Can you work these out from the model? Positions are in its coordinate system, mm. A direction names the side the tool comes from. Give positions to 0.01 mm unless a question says otherwise; leave off trailing zeros. Write each loop counter-clockwise with the first axis right and the second up, starting at its lowest first coordinate (ties: lowest second). Pieces come first, ordered by that corner, then holes.
1. If I drill on probe 1 along X at (y, z) = (1.2, 58); probe 2 along Z at (x, y) = (-8, 2.4); probe 3 along Z at (x, y) = (41, 1.75), over which ranges is the centre line in solid material (lowest first)?
2. Suppose I cut it at A-A (x = 39). Please give me the cut outline in (y, z) (3 decimals).
3. Suppose I cut it at B-B (y = 2). Give the number of separate pieces and of enclosed holes in the cut face, and give its area (3 significant figures).
4. Suppose I cut it at C-C (z = 26). Please give me the cut outline in (x, y) (3 decimals).
5. On a 3-axis mill with a long thin cutter (end or side, diameter ignored), from which of +Z, -Z, +X, -X, +Y, -Y can I reach the whole of each face in a straight line? I mean faces 1 (the cylindrical face through (0.71, 1.565, 124.636)), 2 (the flat face through (-97.4, 1.6, 23.5)), 3 (the flat face through (97.94, 1.57, 23.25)), 4 (the flat face through (91.042, 1.565, 82.953)), 5 (the cylindrical face through (118.74, 1.61, 1.81)). Say none if no direction works.
6. I'm going to push flat-ended pins straight in: pin 1 (1 mm diameter, centred on y = 2.5, z = 50.5, fed in from -X); pin 2 (4 mm diameter, centred on x = -61.5, z = 40, fed in from -Y); pin 3 (1 mm diameter, centred on x = 36.5, y = 1, fed in from +Z). Where does each tip first touch, or does it pass through?
7. Suppose I cut it at D-D (x = -33). Please give me the cut outline in (y, z) (3 decimals), and give its area (3 significant figures).
8. Thinking about a two-plate mould opening in Z: for faces 6 (the flat face through (-41.28, 1.57, 87.93)), 7 (the flat face through (18, 3.175, 76)), 8 (the cylindrical face through (118.84, 1.61, 131.44)), 9 (the cylindrical face through (-118.74, 1.61, 1.81)), which applies, pulls with the +Z half, pulls with the -Z half, needs draft (parallel to the pull), parting line crosses it, or undercut?
```python
from build123d import *

# Parameters (mm, degrees)
BOSS_EXTRUDE1_DEPTH = 3.175
FILLET1_R           = 6.35
FILLET2_R           = 6.35


with BuildPart() as part:
    # Sketch1 → Boss-Extrude1 (new body)
    with BuildSketch(Plane(origin=(0, 0, 0), x_dir=(1, 0, 0), z_dir=(0, 1, 0))):
        with BuildLine():
            Line((-120.65, 0), (120.65, 0))
            Line((120.65, 0), (120.65, -12.7))
            Line((120.65, -12.7), (65.976752043, -38.1))
            Line((65.976752043, -38.1), (120.65, -63.5))
            Line((120.65, -63.5), (120.65, -76.2))
            Line((120.65, -76.2), (79.645064032, -95.25))
            Line((79.645064032, -95.25), (120.65, -114.3))
            Line((120.65, -114.3), (120.65, -133.35))
            Line((120.65, -133.35), (50.8, -133.35))
            ThreePointArc((50.8, -133.35), (0, -124.634097937), (-50.8, -133.35))
            Line((-50.8, -133.35), (-120.65, -133.35))
            Line((-120.65, -133.35), (-120.65, -114.3))
            Line((-120.65, -114.3), (-79.645064032, -95.25))
            Line((-79.645064032, -95.25), (-120.65, -76.2))
            Line((-120.65, -76.2), (-120.65, -63.5))
            Line((-120.65, -63.5), (-65.976752043, -38.1))
            Line((-65.976752043, -38.1), (-120.65, -12.7))
            Line((-120.65, -12.7), (-120.65, 0))
        make_face()
        Polygon((-111.711303819, -6.35), (111.711303819, -6.35), (0, -58.248638237), align=None, mode=Mode.SUBTRACT)
        Polygon((-58.441082652, -41.600907842), (-119.246973209, -69.85), (-72.109394642, -91.749092158), (-11.303504085, -63.5), align=None, mode=Mode.SUBTRACT)
        Polygon((11.303504085, -63.5), (58.441082652, -41.600907842), (119.246973209, -69.85), (72.109394642, -91.749092158), align=None, mode=Mode.SUBTRACT)
        with BuildLine():
            Line((-104.877147824, -117.475), (0, -68.751361763))
            Line((0, -68.751361763), (104.877147824, -117.475))
            Line((104.877147824, -117.475), (62.737522787, -117.475))
            ThreePointArc((62.737522787, -117.475), (0, -105.584097937), (-62.737522787, -117.475))
            Line((-62.737522787, -117.475), (-104.877147824, -117.475))
        make_face(mode=Mode.SUBTRACT)
    extrude(amount=BOSS_EXTRUDE1_DEPTH)

    # Fillet1
    fillet1_edges = [part.edges().sort_by_distance(p)[0] for p in [
        (104.877147824, 1.5875, 117.475),
        (0, 1.5875, 68.751361763),
        (-104.877147824, 1.5875, 117.475),
        (-62.737522787, 1.5875, 117.475),
        (-111.711303819, 1.5875, 6.35),
        (0, 1.5875, 58.248638237),
        (111.711303819, 1.5875, 6.35),
        (-11.303504085, 1.5875, 63.5),
        (-58.441082652, 1.5875, 41.600907842),
        (-119.246973209, 1.5875, 69.85),
        (-72.109394642, 1.5875, 91.749092158),
        (11.303504085, 1.5875, 63.5),
        (72.109394642, 1.5875, 91.749092158),
        (119.246973209, 1.5875, 69.85),
        (58.441082652, 1.5875, 41.600907842),
    ]]
    fillet(fillet1_edges, radius=FILLET1_R)

    # Fillet2
    fillet2_edges = [part.edges().sort_by_distance(p)[0] for p in [
        (120.65, 1.5875, 12.7),
        (65.976752043, 1.5875, 38.1),
        (120.65, 1.5875, 63.5),
        (120.65, 1.5875, 76.2),
        (79.645064032, 1.5875, 95.25),
        (120.65, 1.5875, 114.3),
        (120.65, 1.5875, 133.35),
        (50.8, 1.5875, 133.35),
        (-50.8, 1.5875, 133.35),
        (-120.65, 1.5875, 133.35),
        (-120.65, 1.5875, 114.3),
        (-79.645064032, 1.5875, 95.25),
        (-120.65, 1.5875, 76.2),
        (-120.65, 1.5875, 63.5),
        (-65.976752043, 1.5875, 38.1),
        (-120.65, 1.5875, 12.7),
        (-120.65, 1.5875, 0),
        (120.65, 1.5875, 0),
    ]]
    fillet(fillet2_edges, radius=FILLET2_R)


solid = part.part
```
Checks:
1. probe 1: x = -108.81 to -93.74, -23.2 to 23.2, 93.74 to 108.81
1. probe 2: z = 0 to 6.35, 54.53 to 72.47, 105.77 to 124.84
1. probe 3: z = 0 to 6.35, 39.2 to 49.7, 77.3 to 87.8, 110.56 to 130.25
2. outline: (0, 0) - (3.175, 0) - (3.175, 6.35) - (0, 6.35) - close; (0, 40.13) - (3.175, 40.13) - (3.175, 50.633) - (0, 50.633) - close; (0, 76.367) - (3.175, 76.367) - (3.175, 86.87) - (0, 86.87) - close; (0, 110.079) - (3.175, 110.079) - (3.175, 129.709) - (0, 129.709) - close
3. separate pieces: 1
3. enclosed holes: 4
3. area: 12,800 mm2
4. outline: (-92.022, 0) - (-69.415, 0) - (-69.415, 3.175) - (-92.022, 3.175) - close; (69.415, 0) - (92.022, 0) - (92.022, 3.175) - (69.415, 3.175) - close
5. face 1: +Z, +Y, -Y
5. face 2: -X, +Y, -Y
5. face 3: +X, +Y, -Y
5. face 4: +Y, -Y
5. face 5: -Z, +X, +Y, -Y
6. pin 1: stops at x = -93.74
6. pin 2: stops at y = 0
6. pin 3: stops at z = 129.19
7. outline: (0, 0) - (3.175, 0) - (3.175, 6.35) - (0, 6.35) - close; (0, 42.918) - (3.175, 42.918) - (3.175, 53.42) - (0, 53.42) - close; (0, 73.58) - (3.175, 73.58) - (3.175, 84.082) - (0, 84.082) - close; (0, 108.79) - (3.175, 108.79) - (3.175, 128.25) - (0, 128.25) - close
7. area: 149 mm2
8. face 6: undercut
8. face 7: needs draft
8. face 8: pulls with the +Z half
8. face 9: pulls with the -Z half
